Geometry: see drawing. Coordinates: mm, zero at the bounding-box minimum. Give positions to 0.01 mm unless a question says otherwise; leave off trailing zeros. Loops run counter-clockwise (first coordinate to the right, second up) from the corner with the lowest first, then second, coordinate; pieces in that order, holes last. Notation, with made-up numbers: M 3.25,-37.75 L 56.25,-37.75 A9 ccw 56.25,-28.75 Z; hole C 79.25,74.25 d11. An arc over 180 degrees is marked long. Put each result on its own line as item: value.
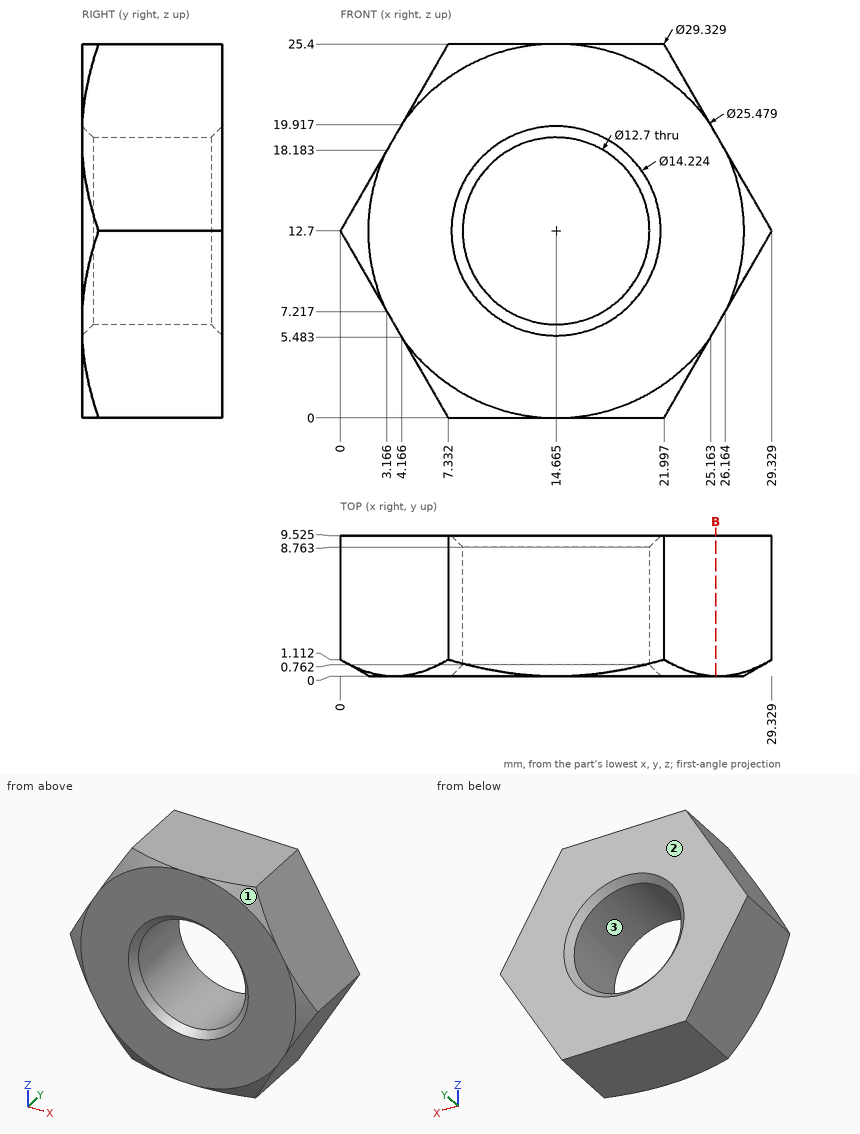
1. Draft query along X for the marked faces 1, 2 and 3. Return one class per face: pulls with the +X half, pulls with the -X half, needs draft (parallel to the pull), parting line crosses it, or undercut.
Found:
face 1: pulls with the +X half
face 2: needs draft
face 3: undercut
2. Material intervals for line 1 (Z direction, x = 14.5, y = 6.25); line 2 (Z direction, x = 10.5, y = 4.75) (1 decimal); line 3 (Z direction, x = 24, y = 5) (1 decimal), sorted ascending. Write a range as from..to.
Found:
line 1: 0..6.35, 19.05..25.4
line 2: 0..7.9, 17.5..25.4
line 3: 3.5..21.9
3. Contact query for flat-ended pins moving along their axis: P1, Ø5, axis at y = 4, z = 22.5, coming from the +X side (1 decimal); P2, Ø4, axis at y = 6.5, z = 17, coming from the -X side. Output: stop coordinate, or through.
Found:
P1: x = 25.1
P2: x = 1.33
4. Section query B-B (x = 25.5). Output: boundary loops of the cut face in (y, z) (1 decimal).
Found:
outline: M 0,6.1 L 9.5,6.1 L 9.5,19.3 L 0,19.3 Z
